Design review of the part built by this model. Coordinates are the model's own, in mm. A direction names the side the tool comes from. Round coordinates to 2 decimals unless told otherwise and drop trailing zeros. Loops run counter-clockwise (first coordinate to the right, second up) from the corner with the lowest first, then second, coordinate; pieces in that order, holes last. Notation, with made-up numbers: M -19.5,75.5 L 3.5,75.5 A16 cw 3.5,91.5 Z; hole C 83,80 d7. An arc over 180 degrees is marked long. Use a Markdown table: item, result.
from build123d import *

# Parameters (mm, degrees)
CROQUIS1_W              = 133.8
CROQUIS1_H              = 30
CROQUIS1_R              = 5
SALIENTE_EXTRUIR1_DEPTH = 60
CROQUIS2_W              = 123.8
CROQUIS2_H              = 50
CORTAR_EXTRUIR1_DEPTH   = 119.130169906
CROQUIS3_R              = 5
CORTAR_EXTRUIR2_DEPTH   = 10


with BuildPart() as part:
    # Croquis1 → Saliente-Extruir1 (new body)
    with BuildSketch(Plane(origin=(0, 0, 0), x_dir=(1, 0, 0), z_dir=(0, 1, 0))):
        with Locations((30.335472139, 9.642857143)):
            Rectangle(CROQUIS1_W, CROQUIS1_H)
        with Locations(Location((-26.564527861, 7.494831092, 0), (0, 0, 270))):
            Circle(CROQUIS1_R, mode=Mode.SUBTRACT)
    extrude(amount=SALIENTE_EXTRUIR1_DEPTH)

    # Croquis2 → Cortar-Extruir1 (cut, through all)
    with BuildSketch(Plane.XY.offset(5.357142857)):
        with Locations((30.335472139, 30)):
            Rectangle(CROQUIS2_W, CROQUIS2_H)
    extrude(amount=-CORTAR_EXTRUIR1_DEPTH, mode=Mode.SUBTRACT)

    # Croquis3 → Cortar-Extruir2 (cut)
    with BuildSketch(Plane(origin=(97.235472139, 0, 0), x_dir=(0, 0, -1), z_dir=(1, 0, 0))):
        with Locations((9.642857143, 30)):
            Circle(CROQUIS3_R)
    extrude(amount=-CORTAR_EXTRUIR2_DEPTH, mode=Mode.SUBTRACT)


solid = part.part
1. Take a section at A-A on y = 30. Give the boundary of the cut face in (x, z), and give its area (3 significant figures).
Check values:
| item | result |
|---|---|
| outline | M -36.56,-24.64 L -31.56,-24.64 L -31.56,5.36 L -36.56,5.36 Z; M 92.24,-24.64 L 97.24,-24.64 L 97.24,-14.64 L 92.24,-14.64 Z; M 92.24,-4.64 L 97.24,-4.64 L 97.24,5.36 L 92.24,5.36 Z |
| area | 250 mm² |
2. Take a section at B-B on x = 35. Give the boundary of the cut face in (y, z).
Check values:
| item | result |
|---|---|
| outline | M 0,-24.64 L 5,-24.64 L 5,5.36 L 0,5.36 Z; M 55,-24.64 L 60,-24.64 L 60,5.36 L 55,5.36 Z |
3. Machinability: for faces 5 (the face through (29, 5, -9)), 6 (the face through (97.235, 30, -16)), which of the approach directions +Z, -Z, +X, -X, +Y, -Y give a long, thin tool a straight path to every point of the face, cutting with its end or side? Answer none if there is none.
Check values:
| item | result |
|---|---|
| face 5 | +Z, -Z |
| face 6 | +Z, -Z, +X, +Y, -Y |
4. Take a section at D-D on z = -19. Give the boundary of the cut face in (x, y).
Check values:
| item | result |
|---|---|
| outline | M -36.56,0 L 97.24,0 L 97.24,60 L -36.56,60 Z; hole M -31.56,5 L 92.24,5 L 92.24,55 L -31.56,55 Z |
5. Wall thickness on line 1 along Y through (x, z) = (10.5, -5.25); line 2 along X through (y, z) = (49, 1); line 3 along X through (y, z) = (26, -8.5): over which ranges is each line inside the solid? List them lowest first. Write a range as from..to.
Check values:
| item | result |
|---|---|
| line 1 | y = 0..5, 55..60 |
| line 2 | x = -36.56..-31.56, 92.24..97.24 |
| line 3 | x = -36.56..-31.56 |
6. Take a section at C-C on y = 23. Give the boundary of the cut face in (x, z).
Check values:
| item | result |
|---|---|
| outline | M -36.56,-24.64 L -31.56,-24.64 L -31.56,5.36 L -36.56,5.36 Z; M 92.24,-24.64 L 97.24,-24.64 L 97.24,5.36 L 92.24,5.36 Z |
7. The part is to be moulded in two halves that separate along Z. For faces 1 (the face through (94.77, 26.958, -5.675)), 2 (the face through (-29.61, 2.46, -11.46)), 3 (the face through (92.235, 24, -9)), 4 (the face through (25, 57, 5.357)), say which applies: pulls with the +Z half, pulls with the -Z half, needs draft (parallel to the pull), parting line crosses it, or undercut.
Check values:
| item | result |
|---|---|
| face 1 | undercut |
| face 2 | undercut |
| face 3 | needs draft |
| face 4 | pulls with the +Z half |
